from build123d import *

# Parameters (mm, degrees)
F0_W          = 210
F0_H          = 225
F1_DEPTH      = 25
F3_DEPTH      = 95
F4_R          = 37.5
F5_DEPTH      = 10
F5_DEPTH_BACK = 127
F6_R          = 40
F7_DEPTH      = 10
F7_DEPTH_BACK = 127
F8_W          = 60
F8_H          = 60
F9_DEPTH      = 10
F10_R         = 10


with BuildPart() as f1:
    # F0 (on Top) → F1 (new body)
    with BuildSketch(Plane.XY):
        with Locations((-1.685321, 68.338609)):
            Rectangle(F0_W, F0_H)
    extrude(amount=F1_DEPTH)

    # F2 (on face) → F3 (join)
    with BuildSketch(Plane.XY.offset(25)):
        with BuildLine():
            Line((-26.685321, 131.838609), (-106.685321, 131.838609))
            Line((-106.685321, 131.838609), (-106.685321, 116.838609))
            Line((-106.685321, 116.838609), (-40.667138, 116.838609))
            ThreePointArc((-40.667138, 116.838609), (-9.174174, 53.349757), (54.314679, 21.856793))
            Line((54.314679, 21.856793), (54.314679, -44.161391))
            Line((54.314679, -44.161391), (69.314679, -44.161391))
            Line((69.314679, -44.161391), (69.314679, 35.838609))
            ThreePointArc((69.314679, 35.838609), (1.432428, 63.956358), (-26.685321, 131.838609))
        make_face()
    extrude(amount=F3_DEPTH)

    # F4 (on face) → F5 (join, two sides)
    with BuildSketch(Plane(origin=(-106.685321, 0, 0), x_dir=(0, -1, 0), z_dir=(-1, 0, 0))) as f5_sk:
        with Locations((-124.338609, 120)):
            Circle(F4_R)
    extrude(amount=F5_DEPTH)
    extrude(f5_sk.sketch, amount=-F5_DEPTH_BACK)

    # F6 (on face) → F7 (join, two sides)
    with BuildSketch(Plane.XZ.offset(44.161391)) as f7_sk:
        with Locations((61.814679, 120)):
            Circle(F6_R)
    extrude(amount=F7_DEPTH)
    extrude(f7_sk.sketch, amount=-F7_DEPTH_BACK)

    # F8 (on face) → F9 (join)
    with BuildSketch(Plane.XY.offset(25)):
        with Locations((-76.685321, -14.161391)):
            Rectangle(F8_W, F8_H)
    extrude(amount=F9_DEPTH)

    # F10
    f10_edges = [f1.edges().sort_by_distance(p)[0] for p in [
        (-46.685321, 15.838609, 30),
    ]]
    fillet(f10_edges, radius=F10_R)


solid = f1.part
Could you check a few things on this model? Use its own coordinates, in mm. A direction names the side the tool comes from. Round coordinates to 2 decimals unless told otherwise and drop trailing zeros. Loops run counter-clockwise (first coordinate to the right, second up) from the corner with the lowest first, then second, coordinate; pieces in that order, holes last. Notation, with made-up numbers: (50, 44) - (98, 44) arc R20 ccw to (98, 73) - close; hole circle Ø3 at (-15.5, 61.5). An arc over 180 degrees is marked (long way). Write item = value, one per line.
1) Imagine slicing it at A-A (x = -95). Please give me the cut outline in (y, z), and give its area (3 significant figures).
Computed:
outline = (-44.16, 0) - (180.84, 0) - (180.84, 25) - (131.84, 25) - (131.84, 83.26) arc R37.5 ccw (long way) to (116.84, 83.26) - (116.84, 25) - (15.84, 25) - (15.84, 35) - (-44.16, 35) - close
area = 11,500 mm2
2) I'm going to push flat-ended pins straight in: P1, Ø16.5, axis at y = -20, z = 65, coming from the -X side; P2, Ø6, axis at y = 54, z = 52.5, coming from the +X side; P3, Ø6, axis at x = 42.5, y = -23, coming from the -Z side; P4, Ø12, axis at x = -64, y = 131.5, coming from the +Z side. Where does each tip first touch, or does it pass through?
Computed:
P1 = 54.31
P2 = 17.54
P3 = 0
P4 = 157.48
3) Imagine slicing it at D-D (z = 75). Please give me the cut outline in (x, y).
Computed:
outline = (-106.69, 116.84) - (-40.67, 116.84) arc R111 ccw to (54.31, 21.86) - (54.31, -44.16) - (69.31, -44.16) - (69.31, 35.84) arc R96 cw to (-26.69, 131.84) - (-106.69, 131.84) - close
4) I need wall thicknesses on line 1 along Y through (x, z) = (11, 120.5); line 2 along Z through (x, y) = (-104, -15); line 3 along X through (y, z) = (123, 83). Which ranges of each line are inside material? Lowest first, please. Write a range as from..to.
Computed:
line_1 = 86.84..161.84
line_2 = 0..35
line_3 = -116.69..20.31
5) Imagine slicing it at C-C (y = -25.5). Please give me the cut outline in (x, z).
Computed:
outline = (-106.69, 0) - (103.31, 0) - (103.31, 25) - (69.31, 25) - (69.31, 80.71) arc R40 ccw (long way) to (54.31, 80.71) - (54.31, 25) - (-46.69, 25) - (-46.69, 35) - (-106.69, 35) - close
6) On a 3-axis mill with a long thin cutter (end or side, diameter ignored), from which of +Z, -Z, +X, -X, +Y, -Y can I reach the whole of each face in a straight line? I mean faces 4 (the flat face through (54.315, -11, 52)), 5 (the cylindrical face through (-9.885, 54.067, 71.835)), 6 (the flat face through (-82, 15.839, 30)), 7 (the flat face through (-46.685, -20, 30)). Say none if no direction works.
Computed:
face_4 = -Y
face_5 = -X, -Y
face_6 = +Z, -X
face_7 = +Z, -Y
7) Imagine slicing it at B-B (z = 141). Please give me the cut outline in (x, y).
Computed:
outline = (-116.69, 93.27) - (20.31, 93.27) - (20.31, 155.41) - (-116.69, 155.41) - close; (27.77, -54.16) - (95.86, -54.16) - (95.86, 82.84) - (27.77, 82.84) - close
8) If we mould it in two halves opening along Z, with no side actions, what happens to faces 1 (the flat face through (61, -54.161, 121)), 2 (the flat face through (-77, -14, 35)), 3 (the flat face through (-27, 37, 25))? For each: pulls with the +Z half, pulls with the -Z half, needs draft (parallel to the pull), parting line crosses it, or undercut.
Computed:
face_1 = needs draft
face_2 = pulls with the +Z half
face_3 = undercut
